```python
from build123d import *

# Parameters (mm, degrees)
SKETCH1_W           = 66.4
SKETCH1_H           = 130
BOSS_EXTRUDE1_DEPTH = 12
SKETCH2_W           = 25
SKETCH2_H           = 45
CUT_EXTRUDE2_DEPTH  = 20
SKETCH3_W           = 25
SKETCH3_H           = 10
BOSS_EXTRUDE2_DEPTH = 12
SKETCH4_R           = 5
BOSS_EXTRUDE4_DEPTH = 12
SKETCH5_W           = 25
SKETCH5_H           = 2
BOSS_EXTRUDE5_DEPTH = 12


with BuildPart() as part:
    # Sketch1 → Boss-Extrude1 (new body)
    with BuildSketch(Plane(origin=(0, 0, 0), x_dir=(1, 0, 0), z_dir=(0, 1, 0))):
        with Locations((33.2, 65)):
            Rectangle(SKETCH1_W, SKETCH1_H)
    extrude(amount=BOSS_EXTRUDE1_DEPTH)

    # Sketch2 → Cut-Extrude2 (cut)
    with BuildSketch(Plane(origin=(0, 12, 0), x_dir=(1, 0, 0), z_dir=(0, 1, 0))):
        with Locations((33.2, 107.5)):
            Rectangle(SKETCH2_W, SKETCH2_H)
    extrude(amount=-CUT_EXTRUDE2_DEPTH, mode=Mode.SUBTRACT)

    # Sketch3 → Boss-Extrude2 (add)
    with BuildSketch(Plane(origin=(0, 12, 0), x_dir=(1, 0, 0), z_dir=(0, 1, 0))):
        with Locations((33.2, 125)):
            Rectangle(SKETCH3_W, SKETCH3_H)
    extrude(amount=-BOSS_EXTRUDE2_DEPTH)



with BuildPart() as body_2:
    # Sketch4 → Boss-Extrude4 (new body)
    with BuildSketch(Plane(origin=(0, 12, 0), x_dir=(1, 0, 0), z_dir=(0, 1, 0))):
        with Locations(Location((33.2, 109, 0), (0, 0, 270))):
            Circle(SKETCH4_R)
    extrude(amount=-BOSS_EXTRUDE4_DEPTH)


with BuildPart() as part_1:
    add(part.part)

    add(body_2.part)  # Boss-Extrude5 merges body 2
    # Sketch5 → Boss-Extrude5 (add)
    with BuildSketch(Plane(origin=(0, 12, 0), x_dir=(1, 0, 0), z_dir=(0, 1, 0))):
        with Locations((33.2, 109)):
            Rectangle(SKETCH5_W, SKETCH5_H)
    extrude(amount=-BOSS_EXTRUDE5_DEPTH)


solid = part_1.part
```
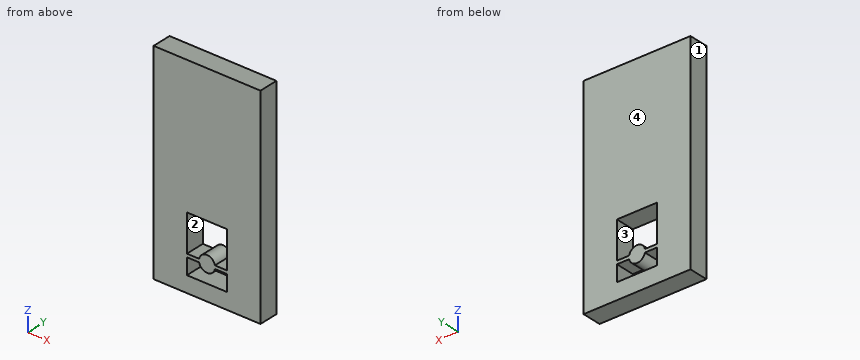
Can you work these out from the model? Positions are in its coordinate system, mm. Face numbers are marked on the shaded views. A direction names the side the tool comes from. Round coordinates to 2 decimals unless told otherwise and drop trailing zeros. Order: outer loops, then holes, each group sorted by start corner. A loop starts at its lowest first (then second) coordinate and runs counter-clockwise, first axis right, second up. Notation, with made-up numbers: (55.5, -7) -> (99.5, -7) arc R36 ccw to (99.5, 29) -> close; hole circle Ø6 at (-28.75, 84). An arc over 180 degrees is marked (long way). Return JSON: item names as keys, results as strings. Group by question number.
1. Which directions (+Z, -Z, +X, -X, +Y, -Y) give clear straight access to the entire face, cutting with the end or side of a thin tool? Please do the marked faces 1 and 2.
2. If we section it at B-B, the plane x = 35: Write out the boundary of the cut face in (y, z).
3. I need wall thicknesses on line 1 (X direction, y = 10, z = -112.5); line 2 (X direction, y = 3, z = -93); line 3 (Z direction, x = 40.5, y = 1.5). Which ranges of each line are inside material? Lowest first, please. Write a range as [from, to].
4. If we section it at A-A, the plane y = 5.25: Write out the boundary of the cut face in (x, z).
5. We'd pull the mould along Z, two halves only. Please class the marked faces 3 and 4: released by +Z, released by -Z, zero draft, split by the parting line, or undercut.
6. Will this pin go through, and if not, where does the flat tip stop? pin 1 (6 mm diameter, centred on x = 36.5, y = 5, fed in from +Z).
Output values:
{
 "1": {"face 1": "+Z, -Z, -X, +Y, -Y", "face 2": "+Y, -Y"},
 "2": {"outline": "(0, -130) -> (12, -130) -> (12, -120) -> (0, -120) -> close; (0, -113.66) -> (12, -113.66) -> (12, -104.34) -> (0, -104.34) -> close; (0, -85) -> (12, -85) -> (12, 0) -> (0, 0) -> close"},
 "3": {"line 1": "[0, 20.7], [29.63, 36.77], [45.7, 66.4]", "line 2": "[0, 20.7], [45.7, 66.4]", "line 3": "[-130, -120], [-110, -108], [-85, 0]"},
 "4": {"outline": "(0, -130) -> (66.4, -130) -> (66.4, 0) -> (0, 0) -> close; hole (20.7, -120) -> (45.7, -120) -> (45.7, -110) -> (38.1, -110) arc R5 cw to (28.3, -110) -> (20.7, -110) -> close; hole (20.7, -108) -> (28.3, -108) arc R5 cw to (38.1, -108) -> (45.7, -108) -> (45.7, -85) -> (20.7, -85) -> close"},
 "5": {"face 3": "undercut", "face 4": "zero draft"},
 "6": {"pin 1": "z = 0"}
}
